from build123d import *

# Parameters (mm, degrees)
BOSS_EXTRUDE1_DEPTH         = 30
BOSS_EXTRUDE1_DEPTH_BACK    = 25
BOSS_EXTRUDE2_DEPTH         = 15
BOSS_EXTRUDE2_DEPTH_BACK    = 15
BOSS_EXTRUDE3_START         = -7
SKETCH5_R                   = 11.5
SKETCH5_R_2                 = 10
BOSS_EXTRUDE3_DEPTH         = 7
SKETCH6_R                   = 2.5
CUT_EXTRUDE1_DEPTH          = 5
M3_TAPPED_HOLE1_D           = 2.5
M3_TAPPED_HOLE1_DEPTH       = 7.5
M3_TAPPED_HOLE1_CSINK_D     = 3.05
M3_TAPPED_HOLE1_CSINK_ANGLE = 90
M3_TAPPED_HOLE1_TIP         = 0.751075774


with BuildPart() as part:
    # Sketch1 → Boss-Extrude1 (new, two sides: drawn at the far end of the back side and taken through both)
    with BuildSketch(Plane.XY.offset(-BOSS_EXTRUDE1_DEPTH_BACK)):
        with BuildLine():
            Line((9.013878189, 15), (0, 15))
            Line((0, 15), (0, 11.5))
            ThreePointArc((0, 11.5), (8.131727984, 8.131727984), (11.5, 0))
            ThreePointArc((11.5, 0), (8.131727984, -8.131727984), (0, -11.5))
            Line((0, -11.5), (0, -15))
            Line((0, -15), (9.013878189, -15))
            ThreePointArc((9.013878189, -15), (15.231429157, -8.617050879), (17.5, 0))
            ThreePointArc((17.5, 0), (15.231429157, 8.617050879), (9.013878189, 15))
        make_face()
        with BuildLine():
            Line((0, 11.5), (0, 15))
            Line((0, 15), (-9.013878189, 15))
            ThreePointArc((-9.013878189, 15), (-17.5, 0), (-9.013878189, -15))
            Line((-9.013878189, -15), (0, -15))
            Line((0, -15), (0, -11.5))
            ThreePointArc((0, -11.5), (-11.5, 0), (0, 11.5))
        make_face()
    extrude(amount=BOSS_EXTRUDE1_DEPTH + BOSS_EXTRUDE1_DEPTH_BACK)

    # Sketch1_23 → Boss-Extrude2 (add, two sides: drawn at the far end of the back side and taken through both)
    with BuildSketch(Plane.XY.offset(-BOSS_EXTRUDE2_DEPTH_BACK)):
        with BuildLine():
            Line((-9.013878189, 15), (-10.828203914, 15))
            ThreePointArc((-10.828203914, 15), (-18.5, 0), (-10.828203914, -15))
            Line((-10.828203914, -15), (-9.013878189, -15))
            ThreePointArc((-9.013878189, -15), (-17.5, 0), (-9.013878189, 15))
        make_face()
        with BuildLine():
            ThreePointArc((18.5, 0), (16.470758519, 8.42402005), (10.828203914, 15))
            Line((10.828203914, 15), (9.013878189, 15))
            ThreePointArc((9.013878189, 15), (15.231429157, 8.617050879), (17.5, 0))
            ThreePointArc((17.5, 0), (15.231429157, -8.617050879), (9.013878189, -15))
            Line((9.013878189, -15), (10.828203914, -15))
            ThreePointArc((10.828203914, -15), (16.470758519, -8.42402005), (18.5, 0))
        make_face()
    extrude(amount=BOSS_EXTRUDE2_DEPTH + BOSS_EXTRUDE2_DEPTH_BACK)

    # Sketch5 → Boss-Extrude3 (add)
    # profile 1 of 3: a face of its own
    with BuildSketch(Plane.XY.offset(30).offset(BOSS_EXTRUDE3_START)):
        with BuildLine():
            ThreePointArc((9.013878189, 15), (0, 17.5), (-9.013878189, 15))
            Line((-9.013878189, 15), (9.013878189, 15))
        make_face()
    # profile 2 of 3: a face of its own
    with BuildSketch(Plane.XY.offset(30).offset(BOSS_EXTRUDE3_START)):
        Circle(SKETCH5_R)
        Circle(SKETCH5_R_2, mode=Mode.SUBTRACT)
    # profile 3 of 3: a face of its own
    with BuildSketch(Plane.XY.offset(30).offset(BOSS_EXTRUDE3_START)):
        with BuildLine():
            ThreePointArc((-9.013878189, -15), (0, -17.5), (9.013878189, -15))
            Line((9.013878189, -15), (-9.013878189, -15))
        make_face()
    extrude(amount=BOSS_EXTRUDE3_DEPTH)

    # Sketch6 → Cut-Extrude1 (cut)
    with BuildSketch(Plane.XY.offset(30)):
        with Locations((5.654398175, 13.080148366)):
            Circle(SKETCH6_R)
        with Locations((8.500541683, -11.436926646)):
            Circle(SKETCH6_R)
        with Locations((-14.154939858, -1.643221721)):
            Circle(SKETCH6_R)
    extrude(amount=-CUT_EXTRUDE1_DEPTH, mode=Mode.SUBTRACT)

    # M3 Tapped Hole1
    with Locations(Plane(origin=(0, -15, 0), x_dir=(-1, 0, 0), z_dir=(0, -1, 0))):
        with Locations((0, 0)):
            CounterSinkHole(M3_TAPPED_HOLE1_D / 2, M3_TAPPED_HOLE1_CSINK_D / 2, depth=M3_TAPPED_HOLE1_DEPTH, counter_sink_angle=M3_TAPPED_HOLE1_CSINK_ANGLE)
            with Locations((0, 0, -(M3_TAPPED_HOLE1_DEPTH + M3_TAPPED_HOLE1_TIP / 2))):  # 118° drill point
                Cone(0, M3_TAPPED_HOLE1_D / 2, M3_TAPPED_HOLE1_TIP, mode=Mode.SUBTRACT)


solid = part.part
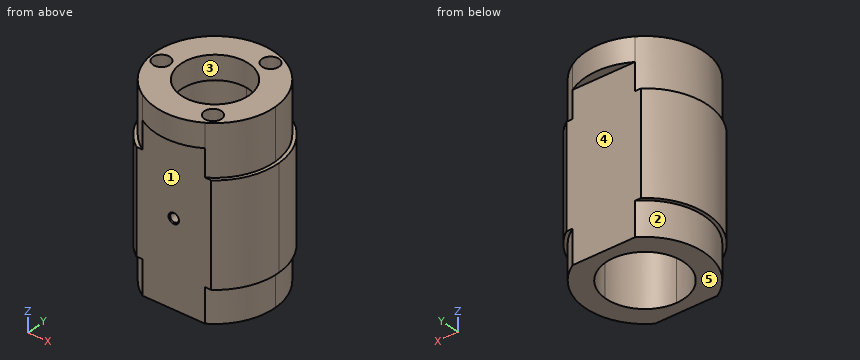
The listing builds one solid part. Answer for the finished solid, in the listing's coordinates (mm). Face numbers are marked on the shaded views. A direction names the side the tool comes from. Round coordinates to 2 decimals unless told otherwise and drop trailing zeros. Loops run counter-clockwise (first coordinate to the right, second up) from the corner with the lowest first, then second, coordinate; pieces in that order, holes last. Notation, with made-up numbers: M -8.5,53.5 L 36.5,53.5 A24 cw 36.5,89.5 Z; hole C -30,79.25 d7. An arc over 180 degrees is marked long. Return JSON: item names as keys, results as strings.
Q1. Find section B-B, the plane x = -6. Determine the outline of the cut face in (y, z).
Results list:
{"outline": "M -16.44,23 L -15,23 L -15,-25 L -9.81,-25 L -9.81,23 L -8,23 L -8,30 L -16.44,30 Z; M 8,23 L 9.81,23 L 9.81,-25 L 15,-25 L 15,23 L 16.44,23 L 16.44,30 L 8,30 Z"}
Q2. Find section D-D, the plane z = 0. Determine the outline of the cut face in (x, y) (3 decimals), plus the area to 3 significant figures.
Results list:
{"outline": "M -10.828,-15 L -1.525,-15 L -1.25,-14.725 L -1.25,-11.432 A11.5 cw long 1.25,-11.432 L 1.25,-14.725 L 1.525,-15 L 10.828,-15 A18.5 ccw 10.828,15 L -10.828,15 A18.5 ccw Z", "area": "548 mm2"}
Q3. Find the intervals of material crossed by line 1 along Y through (x, z) = (0, 26); line 2 along Z through (x, y) = (-11, 14); line 3 along Y through (x, z) = (10.5, -1), in increasing order. Write a range as from..to.
Results list:
{"line 1": "y = -17.5..-10, 10..17.5", "line 2": "z = -15..15", "line 3": "y = -15..-4.69, 4.69..15"}
Q4. Each of these flat-tipped pins is pushed along its axis until it touches: pin 1 Ø2 at (x, z) = (0, 0) entering from -Y; pin 2 Ø5 at (x, z) = (-1.5, -5) entering from -Y; pin 3 Ø3 at (y, z) = (4, -11) entering from -X; pin 4 Ø4 at (x, y) = (-6, -4.5) entering from -Z. Where does it stop, or does it pass through?
Results list:
{"pin 1": "stops at y = 11.46", "pin 2": "stops at y = -15", "pin 3": "stops at x = -18.33", "pin 4": "passes through"}
Q5. Find section A-A, the plane z = -16.5. Determine the outline of the cut face in (x, y).
Results list:
{"outline": "M -9.01,-15 L 9.01,-15 A17.5 ccw 9.01,15 L -9.01,15 A17.5 ccw Z; hole C 0,0 d23"}
Q6. Find section C-C, the plane y = 7. Determine the outline of the cut face in (x, z), plus the area to 3 significant figures.
Results list:
{"outline": "M -17.12,-15 L -16.04,-15 L -16.04,-25 L -9.12,-25 L -9.12,23 L -7.14,23 L -7.14,30 L -16.04,30 L -16.04,15 L -17.12,15 Z; M 7.14,23 L 9.12,23 L 9.12,-25 L 16.04,-25 L 16.04,-15 L 17.12,-15 L 17.12,15 L 16.04,15 L 16.04,30 L 7.14,30 Z", "area": "854 mm2"}
Q7. The mould has two halves that part along X. Classify the marked faces 1, 2 and 3: released by +X, released by -X, zero draft, split by the parting line, or undercut.
Results list:
{"face 1": "zero draft", "face 2": "released by -X", "face 3": "undercut"}
Q8. Which of the six approach directions +Z, -Z, +X, -X, +Y, -Y give full straight-line access (tool end or side, diameter ignored) to the marked faces 4 and 5?
Results list:
{"face 4": "-Z, +X, -X, +Y", "face 5": "-Z, +X, -X, +Y, -Y"}
